Autodesk Inventor part; units mm, degrees
ref_plane "YZ Plane" through (0, 0, 0) normal (1, 0, 0) x (0, 1, 0)
ref_plane "XZ Plane" through (0, 0, 0) normal (0, 1, 0) x (-1, 0, 0)
ref_plane "XY Plane" through (0, 0, 0) normal (0, 0, 1) x (1, 0, 0)
sketch "Sketch3" plane through (0, 0, 0) normal (0, 0, 1) x (1, 0, 0)
  line L0 (0, 0) -> (60, 0)
  line L1 (60, 0) -> (60, 100)
  line L2 (60, 100) -> (0, 100)
  line L3 (0, 100) -> (0, 0)
  dimension "d6" = 60
  dimension "d7" = 100
extrude "Extrusion1" add sketch "Sketch3" along normal blind 25
sketch "Sketch4" plane through (0, 0, 0) normal (0, -1, 0) x (1, 0, 0)
  line L0 (60, 0) -> (0, 0)
  line L1 (5, 0) -> (5, 5)
  line L2 (5, 5) -> (28, 5)
  line L3 (28, 5) -> (28, 6)
  line L4 (28, 6) -> (32, 6)
  line L5 (32, 6) -> (32, 5)
  line L6 (32, 5) -> (55, 5)
  line L7 (55, 5) -> (55, 0)
  line L8 (55, 0) -> (5, 0)
  line L9 (0, 0) -> (0, 25)
  dimension "d14" = 5
  dimension "d15" = 23
  dimension "d16" = 1
  dimension "d17" = 4
  dimension "d18" = 1
  dimension "d19" = 23
  dimension "d20" = 5
  dimension "d21" = 5
extrude "Extrusion2" cut sketch "Sketch4" against normal through all
sketch "Sketch5" plane through (0, 0, 25) normal (0, 0, 1) x (1, 0, 0)
  line L0 (0, 0) -> (60, 0)
  line L1 (0, 100) -> (0, 0)
  point P0 (47, 15)
  point P1 (47, 50)
  point P2 (47, 85)
  point P3 (13, 15)
  point P4 (13, 50)
  point P5 (13, 85)
  dimension "d24" = 15
  dimension "d25" = 47
  dimension "d28" = 35
  dimension "d31" = 34
hole "Hole1" at (47, 15, 25) at (47, 50, 25) at (47, 85, 25) at (13, 15, 25) at (13, 50, 25) at (13, 85, 25) direction (0, 0, -1) diameter 6.4 end through all counterbore diameter 11 counterbore depth 6
sketch "Sketch6" plane through (0, 0, 25) normal (0, -1, 0) x (1, 0, 0)
  line L0 (0, 0) -> (60, 0)
  line L1 (0, -25) -> (0, 0)
  point P0 (20, -10)
  point P1 (40, -10)
  dimension "d41" = 10
  dimension "d42" = 10
  dimension "d43" = 20
  dimension "d44" = 20
hole "Hole2" at (20, 0, 15) at (40, 0, 15) direction (0, 1, 0) diameter 6.917 depth 15 tip angle 118
sketch "Sketch7" plane through (0, 0, 25) normal (0, 0, 1) x (1, 0, 0)
  line L0 (30, 13) -> (30, 57) construction
  line L1 (33, 13) -> (33, 57)
  line L2 (27, 57) -> (27, 13)
  arc A0 (27, 13) -> (33, 13) centre (30, 13) ccw
  arc A1 (33, 57) -> (27, 57) centre (30, 57) ccw
  line L3 (0, 0) -> (60, 0)
  point P0 (30, 35)
  dimension "d52" = 44
  dimension "d53" = 6
  dimension "d54" = 30
  dimension "d55" = 13
extrude "Extrusion3" cut sketch "Sketch7" against normal through all
chamfer "Chamfer2" distance 2 angle 45 3 edges at (0, 50, 25) (30, 100, 25) (60, 50, 25)
Source: CAD feature listing. Evaluate the final solid. Frame: model axes, mm. A direction names the side the tool comes from. Round coordinates to 2 decimals unless told otherwise and drop trailing zeros. Order: outer loops, then holes, each group sorted by start corner. A loop starts at its lowest first (then second) coordinate and runs counter-clockwise, first axis right, second up. Notation, with made-up numbers: (61, 70) -> (69, 70) arc R25 ccw to (69, 83) -> close; hole circle Ø7 at (38, 72). An arc over 180 degrees is marked (long way). One line per item, written item: value. Start each with the question number.
Q1. Pin query (flat end, axial travel): pin 1 (1.5 mm diameter, centred on y = 87, z = 12, fed in from -X); pin 2 (6.5 mm diameter, centred on x = 13, y = 15, fed in from +Z); pin 3 (6 mm diameter, centred on x = 23, y = 54.5, fed in from -Z); pin 4 (4 mm diameter, centred on x = 13, y = 50, fed in from +Z) (1 decimal). Return the tip coordinate at first contact, or that it passes through.
Q2. Section query B-B (z = 7.75). Return the cut outline in (x, y).
Q3. Section query A-A (x = 30). Return the cut outline in (y, z).
Q4. Section query C-C (y = 50). Give the number of separate pieces and of enclosed holes in the cut face, plus the area to 3 significant figures.
Q5. Access query for faces 3 (the cylindrical face through (18.37, 16.19, 21.96)), 4 (the cylindrical face through (19.848, 7.605, 18.455)), 5 (the cylindrical face through (30, 10, 15)). Directions: +Z, -Z, +X, -X, +Y, -Y. A direction counts if a zero-diameter tool reaches every point of the face in a straight line with its end or side. Return the directions, or none.
Q6. Material intervals for probe 1 along Y at (x, z) = (47, 11.5); probe 2 along X at (y, z) = (15, 8.5); probe 3 along X at (y, z) = (4.75, 15), sorted ascending.
Q7. Draft query along X for faces 1 (the flat face through (30, 100, 14)), 2 (the cylindrical face through (12.758, 90.495, 21.958)). Return one class per face: pulls with the +X half, pulls with the -X half, needs draft (parallel to the pull), parting line crosses it, or undercut.
Findings below:
1. pin 1: x = 0
1. pin 2: z = 19
1. pin 3: z = 5
1. pin 4: through
2. outline: (0, 0) -> (60, 0) -> (60, 100) -> (0, 100) -> close; hole circle Ø6.4 at (13, 15); hole circle Ø6.4 at (13, 50); hole circle Ø6.4 at (13, 85); hole (27, 13) arc R3 ccw to (33, 13) -> (33, 57) arc R3 ccw to (27, 57) -> close; hole circle Ø6.4 at (47, 15); hole circle Ø6.4 at (47, 50); hole circle Ø6.4 at (47, 85)
3. outline: (0, 6) -> (10, 6) -> (10, 25) -> (0, 25) -> close; (60, 6) -> (100, 6) -> (100, 23) -> (98, 25) -> (60, 25) -> close
4. separate pieces: 4
4. enclosed holes: 0
4. area: 815 mm²
5. face 3: +Z
5. face 4: -Y
5. face 5: +Z, -Z
6. probe 1: 0 to 11.8, 18.2 to 46.8, 53.2 to 81.8, 88.2 to 100
6. probe 2: 0 to 9.8, 16.2 to 27, 33 to 43.8, 50.2 to 60
6. probe 3: 0 to 16.54, 23.46 to 36.54, 43.46 to 60
7. face 1: needs draft
7. face 2: undercut
